from build123d import *

# Parameters (mm, degrees)
SKETCH1_W              = 82.55
SKETCH1_H              = 31.75
PLATE_DEPTH            = 4
F_10_CLEARANCE_HOLE1_D = 5.1054
LOAD_CELL_CUTOUT_REACH = 46.94
FILLET1_R              = 3.175
SKETCH8_W              = 25.4
SKETCH8_H              = 3.175
CABLE_CUTOUT_DEPTH     = 53.227273766


with BuildPart() as part:
    # Sketch1 → Plate (new, symmetric)
    with BuildSketch(Plane(origin=(0, 0, 0), x_dir=(1, 0, 0), z_dir=(0, 1, 0))):
        Rectangle(SKETCH1_W, SKETCH1_H)
    extrude(amount=PLATE_DEPTH, both=True)

    # #10 Clearance Hole1 (through all)
    with Locations(Plane(origin=(0, 4, 0), x_dir=(1, 0, 0), z_dir=(0, 1, 0))):
        with Locations((-36.5125, 11.1125), (36.5125, 11.1125), (36.5125, -11.1125), (-36.5125, -11.1125), (0, -11.1125), (0, 11.1125)):
            Hole(F_10_CLEARANCE_HOLE1_D / 2)

    # Sketch4 → Load Cell Cutout (cut, up to next)
    with BuildSketch(Plane(origin=(0, 4, 0), x_dir=(1, 0, 0), z_dir=(0, 1, 0)), mode=Mode.PRIVATE) as load_cell_cutout_sk1:
        with BuildLine():
            Line((-11.215130837, 6.927542495), (-5.146572344, 5.008))
            Line((-5.146572344, 5.008), (0.508, 5.008))
            Line((0.508, 5.008), (0.508, -5.008))
            Line((0.508, -5.008), (-5.146572344, -5.008))
            Line((-5.146572344, -5.008), (-11.215130837, -6.927542495))
            ThreePointArc((-11.215130837, -6.927542495), (-35.233, 0), (-11.215130837, 6.927542495))
        make_face()
    load_cell_cutout_tool1 = extrude(load_cell_cutout_sk1.sketch, amount=-LOAD_CELL_CUTOUT_REACH, mode=Mode.PRIVATE) & part.part
    load_cell_cutout = load_cell_cutout_tool1.solids().sort_by_distance((-19.247543, 4, 0))[0]
    add(load_cell_cutout, mode=Mode.SUBTRACT)

    # Cutout Mirror: Load Cell Cutout across plane
    add(load_cell_cutout.mirror(Plane(origin=(0, 0, 0), x_dir=(0, 0, 1), z_dir=(1, 0, 0))), mode=Mode.SUBTRACT)

    # Fillet1
    fillet1_edges = [part.edges().sort_by_distance(p)[0] for p in [
        (-11.215130837, 0, 6.927542495),
        (-11.215130837, 0, -6.927542495),
        (11.215130837, 0, -6.927542495),
        (11.215130837, 0, 6.927542495),
    ]]
    fillet(fillet1_edges, radius=FILLET1_R)

    # Sketch8 → Cable Cutout (cut, through all)
    with BuildSketch(Plane.XY.offset(15.875)):
        with Locations((0, 2.4125)):
            Rectangle(SKETCH8_W, SKETCH8_H)
    extrude(amount=-CABLE_CUTOUT_DEPTH, mode=Mode.SUBTRACT)


solid = part.part
Geometry: final body of the model. Coordinates: model frame, mm. A direction names the side the tool comes from. Coordinates: 2 decimals unless noted, no trailing zeros. Loops run counter-clockwise (first coordinate to the right, second up) from the corner with the lowest first, then second, coordinate; pieces in that order, holes last. Notation, with made-up numbers: (58.25, 4.5) - (114.25, 4.5) arc R32 cw to (114.25, 38.5) - close; hole circle Ø5 at (37.5, 10). An arc over 180 degrees is marked (long way). Put each result on its own line as item: value. Start each with the question number.
Q1. Set-up query: faces 1 (the flat face through (12.7, 2, -12)), 2 (the flat face through (36, 4, 0)), 3 (the flat face through (-7.62, -1.55, 5.79)). Return all of +Z, -Z, +X, -X, +Y, -Y with unobstructed straight access to the full face (end or side cutting, diameter ignored); none if empty.
Q2. Cut plane A-A, the plane x = 0. Return loops of the section in (y, z) (3 decimals), and give its area (3 significant figures).
Q3. Line query: line 1 (Z direction, x = 0, y = -2.65) (3 decimals); line 2 (X direction, y = 1.75, z = -12) (3 decimals); line 3 (X direction, y = 2.75, z = -14) (3 decimals). Output: solid intervals per line, ascending.
Q4. Pin query (flat end, axial travel): pin 1 Ø8.5 at (x, z) = (-5, 11.5) entering from +Y (3 decimals). Return the tip coordinate at first contact, or that it passes through.
Q5. Cut plane D-D, the plane y = -2. Give the number of separate pieces and of enclosed holes in the cut face, and give its area (3 significant figures).
Q6. Cut plane C-C, the plane x = -18. Return loops of the section in (y, z) (3 decimals).
Q7. Cut plane B-B, the plane z = 0. Return loops of the section in (x, y) (3 decimals).
Filled sheet:
1. face 1: +Z, -Z, +Y
1. face 2: +Z, -Z, +X, -X, +Y
1. face 3: +Y, -Y
2. outline: (-4, -15.875) - (0.825, -15.875) - (0.825, -13.665) - (-4, -13.665) - close; (-4, -8.56) - (0.825, -8.56) - (0.825, -5.008) - (-4, -5.008) - close; (-4, 5.008) - (0.825, 5.008) - (0.825, 8.56) - (-4, 8.56) - close; (-4, 13.665) - (0.825, 13.665) - (0.825, 15.875) - (-4, 15.875) - close
2. area: 55.6 mm²
3. line 1: -15.875 to -13.665, -8.56 to -5.008, 5.008 to 8.56, 13.665 to 15.875
3. line 2: -41.275 to -38.906, -34.119 to -27.246, -17.204 to -12.7, 12.7 to 17.204, 27.246 to 34.119, 38.906 to 41.275
3. line 3: -41.275 to -12.7, 12.7 to 41.275
4. pin 1: y = 0.825
5. separate pieces: 1
5. enclosed holes: 7
5. area: 1,220 mm²
6. outline: (-4, -15.875) - (4, -15.875) - (4, -12.303) - (-4, -12.303) - close; (-4, 12.303) - (4, 12.303) - (4, 15.875) - (-4, 15.875) - close
7. outline: (-41.275, -4) - (-35.233, -4) - (-35.233, 4) - (-41.275, 4) - close; (35.233, -4) - (41.275, -4) - (41.275, 4) - (35.233, 4) - close
